Autodesk Inventor part; units mm, degrees
ref_plane "YZ Plane" through (0, 0, 0) normal (1, 0, 0) x (0, 1, 0)
ref_plane "XZ Plane" through (0, 0, 0) normal (0, 1, 0) x (-1, 0, 0)
ref_plane "XY Plane" through (0, 0, 0) normal (0, 0, 1) x (1, 0, 0)
sketch "Skizze2" plane through (0, 0, 0) normal (0, 1, 0) x (-1, 0, 0)
  circle A0 centre (0, 0) radius 75
  line L0 (-102.5, -275) -> (102.5, -275)
  line L1 (102.5, -275) -> (102.5, 275)
  line L2 (102.5, 275) -> (-102.5, 275)
  line L3 (-102.5, 275) -> (-102.5, -275)
  line L4 (-102.5, -275) -> (102.5, 275) construction
  line L5 (102.5, -275) -> (-102.5, 275) construction
  dimension "d8" = 150
  dimension "d9" = 205
  dimension "d10" = 550
extrude "Extrusion1" add sketch "Skizze2" along normal blind 15
sketch "Skizze3" plane through (0, 0, 0) normal (0, -1, 0) x (1, 0, 0)
  line L0 (-92.5, -265) -> (92.5, -265)
  line L1 (92.5, -265) -> (92.5, 265)
  line L2 (92.5, 265) -> (-92.5, 265)
  line L3 (-92.5, 265) -> (-92.5, -265)
  line L4 (-92.5, -265) -> (92.5, 265) construction
  line L5 (92.5, -265) -> (-92.5, 265) construction
  line L6 (-102.5, -275) -> (-102.5, 275)
  line L7 (102.5, 275) -> (102.5, -275)
  point P0 (0, 0)
  dimension "d13" = 185
  dimension "d14" = 530
  dimension "d86" = 205
hole "Bohrung1" at (92.5, 0, -265) at (-92.5, 0, -265) at (-92.5, 0, 265) at (92.5, 0, 265) direction (0, 1, 0) diameter 4.917 end through all
sketch "Skizze6" plane through (0, 0, 0) normal (0, -1, 0) x (1, 0, 0)
  line L0 (99, 275) -> (99, -275)
  line L1 (102.5, 275) -> (102.5, -275)
  line L2 (96.5, 275) -> (96.5, -275)
  line L3 (-99, -275) -> (-99, 275)
  line L4 (-96.5, -275) -> (-96.5, 275)
  line L5 (102.5, -275) -> (-102.5, -275)
  line L6 (96.5, -275) -> (99, -275)
  line L7 (-96.5, -275) -> (-99, -275)
  line L8 (-102.5, 275) -> (102.5, 275)
  line L9 (-96.5, 275) -> (-99, 275)
  line L10 (99, 275) -> (96.5, 275)
  line L11 (-102.5, -275) -> (-102.5, 275)
  point P0 (0, 0)
  point P1 (99, 275)
  point P2 (96.5, 275)
  dimension "d68" = 2.5
  dimension "d70" = 2.5
  dimension "d84" = 198
  dimension "d85" = 99
extrude "Extrusion2" cut sketch "Skizze6" against normal blind 2.5 contours L0 L5 L2 L8 | L4 L5 L3 L8
sketch "Skizze7" plane through (0, 0, 0) normal (0, -1, 0) x (1, 0, 0)
  line L0 (-80, -20) -> (80, -20)
  line L1 (80, -20) -> (80, 20)
  line L2 (80, 20) -> (-80, 20)
  line L3 (-80, 20) -> (-80, -20)
  line L4 (-80, -20) -> (80, 20) construction
  line L5 (80, -20) -> (-80, 20) construction
  point P0 (0, 0)
  dimension "d74" = 160
  dimension "d75" = 40
hole "Bohrung6" at (-80, 0, 20) at (-80, 0, -20) at (80, 0, -20) at (80, 0, 20) direction (0, 1, 0) diameter 8 end through all
sketch "Skizze8" plane through (0, 0, 0) normal (0, -1, 0) x (1, 0, 0)
  line L0 (-62.5, -206) -> (62.5, -206)
  line L1 (62.5, -206) -> (62.5, 206)
  line L2 (62.5, 206) -> (-62.5, 206)
  line L3 (-62.5, 206) -> (-62.5, -206)
  line L4 (-62.5, -206) -> (62.5, 206) construction
  line L5 (62.5, -206) -> (-62.5, 206) construction
  line L6 (-26.5, -206) -> (26.5, -206)
  line L7 (26.5, -206) -> (26.5, 206)
  line L8 (26.5, 206) -> (-26.5, 206)
  line L9 (-26.5, 206) -> (-26.5, -206)
  line L10 (-26.5, -206) -> (26.5, 206) construction
  line L11 (26.5, -206) -> (-26.5, 206) construction
  point P0 (0, 0)
  dimension "d87" = 125
  dimension "d88" = 412
  dimension "d89" = 53
  dimension "d90" = 412
hole "Bohrung7" at (-62.5, 0, 206) at (-26.5, 0, 206) at (26.5, 0, 206) at (62.5, 0, 206) at (62.5, 0, -206) at (26.5, 0, -206) at (-26.5, 0, -206) at (-62.5, 0, -206) direction (0, 1, 0) diameter 4.917 end through all
sketch "Skizze9" plane through (0, 0, 0) normal (0, -1, 0) x (1, 0, 0)
  line L0 (-44.5, -245) -> (44.5, -245)
  line L1 (44.5, -245) -> (44.5, 245)
  line L2 (44.5, 245) -> (-44.5, 245)
  line L3 (-44.5, 245) -> (-44.5, -245)
  line L4 (-44.5, -245) -> (44.5, 245) construction
  line L5 (44.5, -245) -> (-44.5, 245) construction
  line L6 (102.5, 275) -> (102.5, -275)
  point P0 (0, 0)
  dimension "d98" = 490
  dimension "d99" = 58
hole "Bohrung8" at (44.5, 0, 245) at (-44.5, 0, 245) at (-44.5, 0, -245) at (44.5, 0, -245) direction (0, 1, 0) diameter 14 end through all
sketch "Skizze10" plane through (0, 0, 0) normal (0, -1, 0) x (1, 0, 0)
  line L0 (-96.5, 275) -> (96.5, 275)
  line L1 (-102.5, -275) -> (-102.5, 275)
  point P0 (0, 0)
  point P1 (0, 235)
  point P2 (0, 259)
  dimension "d107" = 40
  dimension "d108" = 102.5
  dimension "d116" = 16
  dimension "d117" = 102.5
hole "Bohrung9" at (0, 0, 235) direction (0, 1, 0) diameter 4.917 end through all
sketch "Skizze11" plane through (0, 0, 0) normal (0, -1, 0) x (1, 0, 0)
  line L0 (-102.5, -275) -> (-102.5, 275)
  line L1 (-96.5, 275) -> (96.5, 275)
  point P0 (0, 0)
  point P1 (0, 259)
  dimension "d118" = 102.5
  dimension "d119" = 16
hole "Bohrung10" at (0, 0, 259) direction (0, 1, 0) diameter 5 end through all
equation "\"d70\" = d68"
properties part number "Grundplatte 2.0"
Work out the finished part from the listing and answer in its coordinate system (mm). Give positions to 0.01 mm unless a question says otherwise; leave off trailing zeros. Write each loop counter-clockwise with the first axis right and the second up, starting at its lowest first coordinate (ties: lowest second). Pieces come first, ordered by that corner, then holes.
(1) The part is cut by section C-C on z = 51. Write down the section's boundary in (x, y).
Final values:
outline: (-102.5, 0) - (-99, 0) - (-99, 2.5) - (-96.5, 2.5) - (-96.5, 0) - (-54.99, 0) - (-54.99, 15) - (-102.5, 15) - close; (54.99, 0) - (96.5, 0) - (96.5, 2.5) - (99, 2.5) - (99, 0) - (102.5, 0) - (102.5, 15) - (54.99, 15) - close
(2) The part is cut by section B-B on y = 9.5. Count the separate pieces of the cut face and the enclosed holes in it, plus the area to 3 significant figures.
Final values:
separate pieces: 1
enclosed holes: 23
area: 94,000 mm2
(3) A flat-ended cylindrical pin translates along its axis: pin 1 Ø4 at (x, z) = (92.5, -265) entering from -Y. Find the tip coordinate at first contact, or state that the pin passes through.
Final values:
pin 1: passes through
(4) The part is cut by section A-A on z = 245. Write down the section's boundary in (x, y).
Final values:
outline: (-102.5, 0) - (-99, 0) - (-99, 2.5) - (-96.5, 2.5) - (-96.5, 0) - (-51.5, 0) - (-51.5, 15) - (-102.5, 15) - close; (-37.5, 0) - (37.5, 0) - (37.5, 15) - (-37.5, 15) - close; (51.5, 0) - (96.5, 0) - (96.5, 2.5) - (99, 2.5) - (99, 0) - (102.5, 0) - (102.5, 15) - (51.5, 15) - close
(5) Straight lines are drawn through the part: line 1 (X direction, y = 1.75, z = -213); line 2 (X direction, y = 9, z = -265); line 3 (Z direction, x = 92.5, y = 7.5). For each, find the intervals that lie inside material, in ascending order.
Final values:
line 1: x = -102.5 to -99, -96.5 to 96.5, 99 to 102.5
line 2: x = -102.5 to -94.96, -90.04 to 90.04, 94.96 to 102.5
line 3: z = -275 to -267.46, -262.54 to 262.54, 267.46 to 275
(6) The part is cut by section D-D on x = -16.5. Write down the section's boundary in (y, z), plus the area to 3 significant figures.
Final values:
outline: (0, -275) - (15, -275) - (15, -73.16) - (0, -73.16) - close; (0, 73.16) - (15, 73.16) - (15, 275) - (0, 275) - close
area: 6,060 mm2
(7) The mould has two halves that part along X. Classify faces 1 (the cylindrical face through (9.764, 7.395, -74.362)), 2 (the flat face through (102.5, 7, 4)), 3 (the flat face through (-1, 7, 275)), 4 (the cylindrical face through (-46.603, 7.605, 238.323)): pulls with the +X half, pulls with the -X half, needs draft (parallel to the pull), parting line crosses it, or undercut.
Final values:
face 1: undercut
face 2: pulls with the +X half
face 3: needs draft
face 4: undercut
